```python
from build123d import *
from build123d.topology import SkipClean

# Parameters (mm, degrees)
SKETCH_1_R      = 20
EXTRUDE_1_DEPTH = 50
EXTRUDE_START   = 5
SKETCH_2_R      = 35
SKETCH_2_R_2    = 20
EXTRUDE_2_DEPTH = 5
SKETCH_3_R      = 16


with BuildPart() as part:
    # 草图1 → 凸台-拉伸1 (new body)
    with BuildSketch(Plane.XY):
        with BuildLine():
            Line((18.260869565, 57.153658174), (122.608695652, 23.814024239))
            ThreePointArc((122.608695652, 23.814024239), (140, 0), (122.608695652, -23.814024239))
            Line((122.608695652, -23.814024239), (18.260869565, -57.153658174))
            ThreePointArc((18.260869565, -57.153658174), (-60, 0), (18.260869565, 57.153658174))
        make_face()
        Circle(SKETCH_1_R, mode=Mode.SUBTRACT)
        with BuildLine():
            Line((50, -6.25), (50, 6.25))
            ThreePointArc((50, 6.25), (54.076635218, 14.306906953), (62.982749931, 15.79479978))
            Line((62.982749931, 15.79479978), (82.982749931, 9.54479978))
            ThreePointArc((82.982749931, 9.54479978), (90, 0), (82.982749931, -9.54479978))
            Line((82.982749931, -9.54479978), (62.982749931, -15.79479978))
            ThreePointArc((62.982749931, -15.79479978), (54.076635218, -14.306906953), (50, -6.25))
        make_face(mode=Mode.SUBTRACT)
    extrude(amount=EXTRUDE_1_DEPTH)

    # 草图2 → 凸台-拉伸2 (add)
    with SkipClean():  # the faces are left unmerged after this step: merging them gives an invalid solid
        with BuildSketch(Plane(origin=(0, 0, 0), x_dir=(-1, 0, 0), z_dir=(0, 0, -1)).offset(EXTRUDE_START)):
            with Locations(Location((0, 0, 0), (0, 0, 180))):
                Circle(SKETCH_2_R)
            Circle(SKETCH_2_R_2, mode=Mode.SUBTRACT)
        extrude_2 = extrude(amount=-EXTRUDE_2_DEPTH)

    # 镜向1: 凸台-拉伸2 across plane
    add(extrude_2.mirror(Plane(origin=(0, 0, 25), x_dir=(1, 0, 0), z_dir=(0, 0, -1))))

    # 切除-扫描1: sweep along a path in 草图6
    with BuildLine(Plane(origin=(0, 0, 25), x_dir=(-1, 0, 0), z_dir=(0, 0, -1))) as sweep_1_path:
        Line((-122.608695652, 23.814024239), (-18.260869565, 57.153658174))
        ThreePointArc((-18.260869565, 57.153658174), (60, 0), (-18.260869565, -57.153658174))
        Line((-18.260869565, -57.153658174), (-122.608695652, -23.814024239))
        ThreePointArc((-122.608695652, -23.814024239), (-140, 0), (-122.608695652, 23.814024239))
    # 草图3 → 切除-扫描1 (sweep, cut)
    with BuildSketch(Plane(origin=(0, 0, 0), x_dir=(-1, 0, 0), z_dir=(0, -1, 0))):
        with Locations((-140, -25)):
            Circle(SKETCH_3_R)
    sweep(path=sweep_1_path.line, mode=Mode.SUBTRACT)


solid = part.part
```
The listing builds one solid part. Answer for the finished solid, in the listing's coordinates (mm). A direction names the side the tool comes from. Give positions to 0.01 mm unless a question says otherwise; leave off trailing zeros. Order: outer loops, then holes, each group sorted by start corner. A loop starts at its lowest first (then second) coordinate and runs counter-clockwise, first axis right, second up. Notation, with made-up numbers: (-32.75, 23) - (0.25, 23) arc R15 cw to (0.25, 46) - close; hole circle Ø11 at (26.5, 31). An arc over 180 degrees is marked (long way). Answer in a Markdown table with one row per item. Add a question column.
Q1. Which of the six approach directions +Z, -Z, +X, -X, +Y, -Y give full straight-line access (tool end or side, diameter ignored) to faces 1 (the cylindrical face through (90, 0, 25)), 2 (the cylindrical face through (-7.587, 34.168, -2.535)), 3 (the flat face through (15, 15, 55))?
Q2. For a pull along X with two mould halves and no side action, classify faces 4 (the cylindrical face through (-7.587, 34.168, 52.535)), 5 (the cylindrical face through (53.971, 14.229, 24.65)), 6 (the flat face through (41, 1, 50)) as released by +X, released by -X, zero draft, split by the parting line, or undercut.
Q3. Find the intervals of material crossed by line 1 along Y through (x, z) = (0, 51); line 2 along X through (y, z) = (1.5, 48); line 3 along Y through (x, z) = (66, 13.5), in increasing order. Write a range as [from, to].
Q4. The part is cut by section B-B (z = 46). Determine the outline of the cut face in (x, y), then the cut area to 3 significant figures.
Q5. Given P1, Ø1, axis at y = -20, z = 25.5, coming from the -X side; P2, Ø1, axis at y = 2.5, z = 11, coming from the +X side; P3, Ø4, axis at y = -1.5, z = 27.5, coming from the +X side, each flat-ended and moving along its own axis, determine where each tip first touches the part or whether it passes through.
Q6. The part is cut by section C-C (z = 31). Determine the outline of the cut face in (x, y), then the cut area to 3 significant figures.
Q7. The part is cut by section A-A (y = 0). Determine the outline of the cut face in (x, z).
Determined:
| question | item | result |
|---|---|---|
| 1 | face 1 | +Z, -Z |
| 1 | face 2 | -Z |
| 1 | face 3 | +Z, +X, -X, +Y, -Y |
| 2 | face 4 | split by the parting line |
| 2 | face 5 | undercut |
| 2 | face 6 | zero draft |
| 3 | line 1 | y = [-35, -20], [20, 35] |
| 3 | line 2 | x = [-59.98, -19.94], [19.94, 50], [89.89, 139.95] |
| 3 | line 3 | y = [-30.22, -14.85], [14.85, 30.22] |
| 4 | outline | (18.26, -57.15) - (122.61, -23.81) arc R25 ccw to (122.61, 23.81) - (18.26, 57.15) arc R60 ccw (long way) to start; hole circle Ø40 at (0, 0); hole (50, -6.25) arc R10 ccw to (62.98, -15.79) - (82.98, -9.54) arc R10 ccw to (82.98, 9.54) - (62.98, 15.79) arc R10 ccw to (50, 6.25) - close |
| 4 | area | 14,600 mm² |
| 5 | P1 | stops at x = -39.45 |
| 5 | P2 | stops at x = 133.07 |
| 5 | P3 | stops at x = 124.58 |
| 6 | outline | (13.75, -43.02) - (118.09, -9.69) arc R10.17 ccw to (118.09, 9.69) - (13.75, 43.02) arc R45.17 ccw (long way) to start; hole circle Ø40 at (0, 0); hole (50, -6.25) arc R10 ccw to (62.98, -15.79) - (82.98, -9.54) arc R10 ccw to (82.98, 9.54) - (62.98, 15.79) arc R10 ccw to (50, 6.25) - close |
| 6 | area | 7,790 mm² |
| 7 | outline | (-60, 0) - (-35, 0) - (-35, -5) - (-20, -5) - (-20, 55) - (-35, 55) - (-35, 50) - (-60, 50) - (-60, 41) arc R16 cw to (-60, 9) - close; (20, -5) - (35, -5) - (35, 0) - (50, 0) - (50, 50) - (35, 50) - (35, 55) - (20, 55) - close; (90, 0) - (140, 0) - (140, 9) arc R16 cw to (140, 41) - (140, 50) - (90, 50) - close |
